Model file for the job. Use its own axes, mm. A direction names the side the tool comes from. Coordinates: 2 decimals unless noted, no trailing zeros. Write each loop counter-clockwise with the first axis right and the second up, starting at its lowest first coordinate (ties: lowest second). Pieces come first, ordered by that corner, then holes. Notation, with made-up numbers: (-22, 45.5) - (-18, 45.5) arc R22 cw to (-18, 79.5) - close; hole circle Ø3 at (74, 86.25). An arc over 180 degrees is marked (long way). Put each result on its own line as item: value. Start each with the question number.
1. Pull direction X, two halves, no side cores. Call faces 1 (the face through (24, 11, -1.25)), 2 (the face through (12, -10, 0)), 3 (the face through (0, -0.4, -0.4)): released by +X, released by -X, zero draft, split by the parting line, or undercut.
2. Saw through at B-B, the plane z = -18. Write the cut outline in (x, y).
3. Which spindle directions (+Z, -Z, +X, -X, +Y, -Y) get a long thin tool onto all of the face, cutting with end or side? Do faces 4 (the face through (50, -10, 0)), 5 (the face through (30, 0, 0)), 6 (the face through (25, -19, 8)). Say none if no direction does.
4. Drop flat-ended pins along their axis: P1, Ø2, axis at x = 31.5, z = -1, coming from the +Y side; P2, Ø3, axis at x = 38, z = 0, coming from the +Y side; P3, Ø2, axis at x = 20.5, y = 5.5, coming from the -Z side. Give the stop position or say it passes through.
5. Saw through at D-D, the plane x = 36. Write the cut outline in (y, z), plus the area to 3 significant figures.
6. Saw through at C-C, the plane z = 0. Write the cut outline in (x, y), plus the area to 3 significant figures.
7. Drill centre lines: L1, parallel to X at y = 13, z = 21; L2, parallel to X at y = -15, z = -5; L3, parallel to X at y = -6, z = 26. Where is each one in solid material? Low to high. Write a range as from..to.
8. Saw through at A-A, the plane y = 4. Write the cut outline in (x, z).
```python
from build123d import *

# Parameters (mm, degrees)
SKETCH2_W          = 2.5
SKETCH2_H          = 34.957041577
CUT_EXTRUDE1_DEPTH = 74.484692283


with BuildPart() as part:
    # Sketch1 → Revolve1 (revolve)
    with BuildSketch(Plane.XY, mode=Mode.PRIVATE) as revolve1_sk:
        Polygon((20, 10), (5, 10), (5, 30), (0, 30), (0, 0), (60, 0), (60, 10), (40, 10), (40, 25), (35, 25), (35, 20), (25, 20), (25, 25), (20, 25), align=None)
    revolve(revolve1_sk.sketch.rotate(Axis((0, 0, 0), (1, 0, 0)), 90), axis=Axis((0, 0, 0), (1, 0, 0)))

    # Sketch2 → Cut-Extrude1 (cut, through all)
    with BuildSketch(Plane(origin=(60, 0, 0), x_dir=(0, 0, -1), z_dir=(1, 0, 0))):
        with Locations((0, 17.478520789)):
            Rectangle(SKETCH2_W, SKETCH2_H)
    extrude(amount=-CUT_EXTRUDE1_DEPTH, mode=Mode.SUBTRACT)


solid = part.part
```
Final values:
1. face 1: zero draft
1. face 2: undercut
1. face 3: released by -X
2. outline: (0, -24) - (5, -24) - (5, 24) - (0, 24) - close; (20, -17.35) - (25, -17.35) - (25, -8.72) - (35, -8.72) - (35, -17.35) - (40, -17.35) - (40, 17.35) - (35, 17.35) - (35, 8.72) - (25, 8.72) - (25, 17.35) - (20, 17.35) - close
3. face 4: +X
3. face 5: +X, -X, +Y
3. face 6: none
4. P1: stops at y = 19.96
4. P2: stops at y = 24.97
4. P3: stops at z = -24.59
5. outline: (0, -1.25) - (0, 1.25) - (24.97, 1.25) arc R25 ccw (long way) to (24.97, -1.25) - close
5. area: 1,900 mm²
6. outline: (0, -30) - (5, -30) - (5, -10) - (20, -10) - (20, -25) - (25, -25) - (25, -20) - (35, -20) - (35, -25) - (40, -25) - (40, -10) - (60, -10) - (60, 0) - (0, 0) - close
6. area: 950 mm²
7. L1: x = 0..5, 20..25, 35..40
7. L2: x = 0..5, 20..40
7. L3: x = 0..5
8. outline: (0, -29.73) - (5, -29.73) - (5, -9.17) - (20, -9.17) - (20, -24.68) - (25, -24.68) - (25, -19.6) - (35, -19.6) - (35, -24.68) - (40, -24.68) - (40, -9.17) - (60, -9.17) - (60, -1.25) - (0, -1.25) - close; (0, 1.25) - (60, 1.25) - (60, 9.17) - (40, 9.17) - (40, 24.68) - (35, 24.68) - (35, 19.6) - (25, 19.6) - (25, 24.68) - (20, 24.68) - (20, 9.17) - (5, 9.17) - (5, 29.73) - (0, 29.73) - close
